Geometry: final body of the model. Coordinates: model frame, mm. A direction names the side the tool comes from. Coordinates: 2 decimals unless noted, no trailing zeros. Order: outer loops, then holes, each group sorted by start corner. A loop starts at its lowest first (then second) coordinate and runs counter-clockwise, first axis right, second up. Notation, with made-up numbers: M 35,-3 L 58,-3 A18 ccw 58,24 Z; hole C 4.5,16.25 d5. An arc over 180 degrees is marked long. Write item = value, one per line. Start each with the question number.
```python
from build123d import *

# Parameters (mm, degrees)
F0_W     = 50.8
F0_H     = 50.8
F1_DEPTH = 330.2
F2_DEPTH = 25.4
F4_D     = 16.66748


with BuildPart() as f1:
    # F0 (on Front) → F1 (new body)
    with BuildSketch(Plane.XZ):
        with BuildLine():
            Line((25.4, 31.75), (-25.4, 31.75))
            ThreePointArc((-25.4, 31.75), (-29.8901280605, 29.8901280605), (-31.75, 25.4))
            Line((-31.75, 25.4), (-31.75, -25.4))
            ThreePointArc((-31.75, -25.4), (-29.8901280605, -29.8901280605), (-25.4, -31.75))
            Line((-25.4, -31.75), (25.4, -31.75))
            ThreePointArc((25.4, -31.75), (29.8901280605, -29.8901280605), (31.75, -25.4))
            Line((31.75, -25.4), (31.75, 25.4))
            ThreePointArc((31.75, 25.4), (29.8901280605, 29.8901280605), (25.4, 31.75))
        make_face()
        Rectangle(F0_W, F0_H, mode=Mode.SUBTRACT)
    extrude(amount=-F1_DEPTH)

    # F0 (on Front) → F2 (join)
    with BuildSketch(Plane.XZ):
        with BuildLine():
            Line((25.4, 31.75), (-25.4, 31.75))
            ThreePointArc((-25.4, 31.75), (-29.8901280605, 29.8901280605), (-31.75, 25.4))
            Line((-31.75, 25.4), (-31.75, -25.4))
            ThreePointArc((-31.75, -25.4), (-29.8901280605, -29.8901280605), (-25.4, -31.75))
            Line((-25.4, -31.75), (25.4, -31.75))
            ThreePointArc((25.4, -31.75), (29.8901280605, -29.8901280605), (31.75, -25.4))
            Line((31.75, -25.4), (31.75, 25.4))
            ThreePointArc((31.75, 25.4), (29.8901280605, 29.8901280605), (25.4, 31.75))
        make_face()
        Rectangle(F0_W, F0_H, mode=Mode.SUBTRACT)
    extrude(amount=F2_DEPTH)

    # F4 (through all)
    with Locations(Plane(origin=(-31.75, 0, 0), x_dir=(0, -1, 0), z_dir=(-1, 0, 0))):
        with Locations((-80.720094915, 0)):
            Hole(F4_D / 2)


solid = f1.part
```
Item 1: Section query A-A on z = 0. Output: boundary loops of the cut face in (x, y).
Item 2: Section query B-B on x = -4.5. Output: boundary loops of the cut face in (y, z), and give its area (3 significant figures).
Item 3: Section query D-D on y = 57. Output: boundary loops of the cut face in (x, z), and give its area (3 significant figures).
Item 4: Draft query along Z for faces 3 (the cylindrical face through (-29.84, 154.89, 29.94)), 4 (the flat face through (31.75, 155, 0)), 5 (the flat face through (0, 155, -25.4)). Return one class per face: pulls with the +Z half, pulls with the -Z half, needs draft (parallel to the pull), parting line crosses it, or undercut.
Item 5: Section query C-C on z = 17.5. Output: boundary loops of the cut face in (x, y), and give its area (3 significant figures).
Item 6: Material intervals for probe 1 along X at (y, z) = (-1.5, 21.5); probe 2 along Y at (x, z) = (-28.5, 5.5), sorted ascending. Write a range as [from, to].
Item 7: Reachability of faces 1 (the flat face through (-25.4, 155, 0)), 2 (the flat face through (-29, 330.2, 0)) from +Z, -Z, +X, -X, +Y, -Y: full face, straight path, thin tool, end or side. Return the list, or none.
Ans:
q1.outline = M -31.75,-25.4 L -25.4,-25.4 L -25.4,72.39 L -31.75,72.39 Z; M -31.75,89.05 L -25.4,89.05 L -25.4,330.2 L -31.75,330.2 Z; M 25.4,-25.4 L 31.75,-25.4 L 31.75,72.39 L 25.4,72.39 Z; M 25.4,89.05 L 31.75,89.05 L 31.75,330.2 L 25.4,330.2 Z
q2.outline = M -25.4,-31.75 L 330.2,-31.75 L 330.2,-25.4 L -25.4,-25.4 Z; M -25.4,25.4 L 330.2,25.4 L 330.2,31.75 L -25.4,31.75 Z
q2.area = 4,520 mm^2
q3.outline = M -31.75,-25.4 A6.35 ccw -25.4,-31.75 L 25.4,-31.75 A6.35 ccw 31.75,-25.4 L 31.75,25.4 A6.35 ccw 25.4,31.75 L -25.4,31.75 A6.35 ccw -31.75,25.4 Z; hole M -25.4,-25.4 L 25.4,-25.4 L 25.4,25.4 L -25.4,25.4 Z
q3.area = 1,420 mm^2
q4.face_3 = pulls with the +Z half
q4.face_4 = needs draft
q4.face_5 = undercut
q5.outline = M -31.75,-25.4 L -25.4,-25.4 L -25.4,330.2 L -31.75,330.2 Z; M 25.4,-25.4 L 31.75,-25.4 L 31.75,330.2 L 25.4,330.2 Z
q5.area = 4,520 mm^2
q6.probe_1 = [-31.75, -25.4], [25.4, 31.75]
q6.probe_2 = [-25.4, 74.46], [86.98, 330.2]
q7.face_1 = +Y, -Y
q7.face_2 = +Z, -Z, +X, -X, +Y
